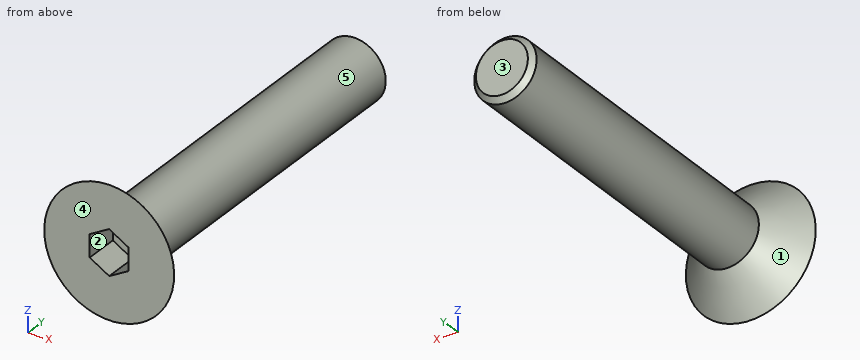
from build123d import *

# Parameters (mm, degrees)
SKETCH_1_R      = 2.5
EXTRUDE_1_DEPTH = 1.3
CHAMFER_1_SIZE  = 1.3
SKETCH_2_R      = 1.2
EXTRUDE_2_DEPTH = 12.7
CHAMFER_2_SIZE  = 0.2


with BuildPart() as part:
    # 草图1 → 凸台-拉伸1 (new body)
    with BuildSketch(Plane(origin=(0, 0, 0), x_dir=(1, 0, 0), z_dir=(0, 1, 0))):
        with Locations(Location((0, 0, 0), (0, 0, 270))):
            Circle(SKETCH_1_R)
        Polygon((0, -0.866025404), (0.75, -0.433012702), (0.75, 0.433012702), (0, 0.866025404), (-0.75, 0.433012702), (-0.75, -0.433012702), align=None, mode=Mode.SUBTRACT)
    extrude(amount=EXTRUDE_1_DEPTH)

    # 倒角1
    # the kernel refuses this chamfer: 1.3 mm, written as the material it takes off along each edge
    with BuildSketch(Plane(origin=(0, 1.3, 0), x_dir=(0, 0, 1), z_dir=(-1, 0, 0))) as chamfer_1_piece_1:
        Polygon((2.5, -CHAMFER_1_SIZE), (2.5 - CHAMFER_1_SIZE, 0), (2.5, 0), align=None)
    revolve(axis=Axis((0, 1.3, 0), (0, 1, 0)), mode=Mode.SUBTRACT)

    # 草图2 → 凸台-拉伸2 (add)
    with BuildSketch(Plane(origin=(0, 1.3, 0), x_dir=(1, 0, 0), z_dir=(0, 1, 0))):
        with Locations(Location((0, 0, 0), (0, 0, 270))):
            Circle(SKETCH_2_R)
    extrude(amount=EXTRUDE_2_DEPTH)

    # 倒角2
    chamfer_2_edges = [part.edges().sort_by_distance(p)[0] for p in [
        (0, 14, -1.2),
    ]]
    chamfer(chamfer_2_edges, length=CHAMFER_2_SIZE)


solid = part.part
Here's how the part is built. I have some questions about the finished solid (model axes, mm). Face numbers are marked on the shaded views. A direction names the side the tool comes from. Coordinates: 2 decimals unless noted, no trailing zeros. Write each loop counter-clockwise with the first axis right and the second up, starting at its lowest first coordinate (ties: lowest second). Pieces come first, ordered by that corner, then holes.
1) If we section it at A-A (z = 0): List the corners of the cut face in (x, y) for me.
Filled in:
outline: (-2.5, 0) - (-0.75, 0) - (-0.75, 1.3) - (0.75, 1.3) - (0.75, 0) - (2.5, 0) - (1.2, 1.3) - (1.2, 13.8) - (1, 14) - (-1, 14) - (-1.2, 13.8) - (-1.2, 1.3) - close
2) I'm going to push a flat-ended pin straight in: pin 1 (2 mm diameter, centred on y = 4.5, z = -1, fed in from +X). Where does the tip first touch, or does it pass through?
Filled in:
pin 1: stops at x = 1.2
3) If we section it at B-B (y = 2): List the corners of the cut face in (x, z) for me.
Filled in:
outline: circle Ø2.4 at (0, 0)
4) Thinking about a two-plate mould opening in Z: for the marked faces 1, 2 and 3, which applies, +Z half, -Z half, draft (parallel to the pull), parting line (faces both ways), or undercut?
Filled in:
face 1: parting line
face 2: undercut
face 3: draft
5) If I drill on line 1 (Z direction, x = 0.9, y = 1); line 2 (Y direction, x = -0.25, z = -0.65); line 3 (Y direction, x = 1.75, z = 0.05), over which ranges is the centre line in solid material (lowest first)?
Filled in:
line 1: z = -1.2 to 1.2
line 2: y = 1.3 to 14
line 3: y = 0 to 0.75
6) Which directions (+Z, -Z, +X, -X, +Y, -Y) give clear straight access to the entire face, cutting with the end or side of a thin tool? Please do the marked faces 4 and 5.
Filled in:
face 4: +Z, -Z, +X, -X, -Y
face 5: +Y
